Autodesk Inventor part; units mm, degrees
ref_plane "YZ Plane" through (0, 0, 0) normal (1, 0, 0) x (0, 1, 0)
ref_plane "XZ Plane" through (0, 0, 0) normal (0, 1, 0) x (-1, 0, 0)
ref_plane "XY Plane" through (0, 0, 0) normal (0, 0, 1) x (1, 0, 0)
sketch "Sketch1" plane through (0, 0, 0) normal (0, 0, 1) x (1, 0, 0)
  line L0 (-15, 12.5) -> (15, 12.5)
  line L1 (15, 12.5) -> (15, -12.5)
  line L2 (15, -12.5) -> (-15, -12.5)
  line L3 (-15, -12.5) -> (-15, 12.5)
  line L4 (-15, 12.5) -> (15, -12.5) construction
  line L5 (15, 12.5) -> (-15, -12.5) construction
  point P0 (0, 0)
  dimension "d0" = 30
  dimension "d1" = 25
extrude "Extrusion1" add sketch "Sketch1" along normal blind 30
sketch "Sketch2" plane through (15, -12.5, 0) normal (1, 0, 0) x (0, 0, -1)
  circle A0 centre (-15.0077, 12.5) radius 7.5
  point P0 (0, 12.5)
  dimension "d4" = 15
extrude "Extrusion2" cut sketch "Sketch2" against normal through all
sketch "Sketch3" plane through (-15, -12.5, 0) normal (0, -1, 0) x (1, 0, 0)
  line L0 (7.5, 23.9638) -> (22.5, 23.9638)
  line L1 (22.5, 23.9638) -> (22.5, 8.9638)
  line L2 (22.5, 8.9638) -> (7.5, 8.9638)
  line L3 (7.5, 8.9638) -> (7.5, 23.9638)
  line L4 (7.5, 23.9638) -> (22.5, 8.9638) construction
  line L5 (22.5, 23.9638) -> (7.5, 8.9638) construction
  point P0 (15, 0)
  point P1 (15, 16.4638)
  dimension "d7" = 15
  dimension "d8" = 15
extrude "Extrusion3" add sketch "Sketch3" along normal blind 25
sketch "Sketch4" plane through (-15, -37.5, 0) normal (0, -1, 0) x (1, 0, 0)
  line L0 (-0.1247, 34.0483) -> (29.8753, 34.0483)
  line L1 (29.8753, 34.0483) -> (29.8753, -0.9517)
  line L2 (29.8753, -0.9517) -> (-0.1247, -0.9517)
  line L3 (-0.1247, -0.9517) -> (-0.1247, 34.0483)
  line L4 (-0.1247, 34.0483) -> (29.8753, -0.9517) construction
  line L5 (29.8753, 34.0483) -> (-0.1247, -0.9517) construction
  point P0 (15, 0)
  point P1 (14.8753, 16.5483)
  dimension "d11" = 30
  dimension "d12" = 35
extrude "Extrusion4" add sketch "Sketch4" along normal blind 30
sketch "Sketch5" plane through (-15.1247, -37.5, -0.9517) normal (-1, 0, 0) x (0, 0, 1)
  circle A0 centre (17.4156, -15.0883) radius 7.5
  point P0 (0.9517, 37.5)
  dimension "d15" = 15
extrude "Extrusion5" add sketch "Sketch5" along normal blind 10
sketch "Sketch6" plane through (14.8753, -37.5, 34.0483) normal (1, 0, 0) x (0, 0, -1)
  circle A0 centre (17.5844, -15.0883) radius 7.5
  circle A1 centre (17.5844, -15.0883) radius 7.5
  point P0 (34.0483, 37.5)
extrude "Extrusion6" add sketch "Sketch6" along normal blind 10
sketch "Sketch7" plane through (-25.1247, -52.5883, 16.4638) normal (-1, 0, 0) x (0, 0, 1)
  line L0 (-17.4156, -14.9117) -> (17.5844, -14.9117)
  circle A0 centre (0, 0) radius 23.0558
  point P0 (-16.4638, 52.5883)
extrude "Extrusion7" add sketch "Sketch7" along normal blind 10
sketch "Sketch8" plane through (24.8753, -52.5883, 16.4638) normal (1, 0, 0) x (0, 0, -1)
  circle A0 centre (0, 0) radius 7.5
  circle A1 centre (0, 0) radius 23.0558
  circle A2 centre (0, 0) radius 23.056
  point P0 (16.4638, 52.5883)
  dimension "d22" = 46.112
extrude "Extrusion8" add sketch "Sketch8" along normal blind 10 contours A0 | A1
sketch "Sketch9" plane through (-15.1247, -37.5, 34.0483) normal (0, 0, 1) x (1, 0, 0)
  line L0 (2.6247, -2.5672) -> (27.6247, -2.5672)
  line L1 (27.6247, -2.5672) -> (27.6247, -27.5672)
  line L2 (27.6247, -27.5672) -> (2.6247, -27.5672)
  line L3 (2.6247, -27.5672) -> (2.6247, -2.5672)
  line L4 (2.6247, -2.5672) -> (27.6247, -27.5672) construction
  line L5 (27.6247, -2.5672) -> (2.6247, -27.5672) construction
  point P0 (15.1247, 37.5)
  point P1 (15.1247, -15.0672)
  dimension "d25" = 25
  dimension "d26" = 25
extrude "Extrusion9" cut sketch "Sketch9" against normal through all
properties part number "Part4f"
The model under review builds one solid part; all positions refer to its coordinate system, in mm. A direction names the side the tool comes from. Coordinates: 2 decimals unless noted, no trailing zeros. Write each loop counter-clockwise with the first axis right and the second up, starting at its lowest first coordinate (ties: lowest second). Pieces come first, ordered by that corner, then holes. Notation, with made-up numbers: (-36, -26) -> (-32, -26) arc R15 cw to (-32, 1) -> close; hole circle Ø7 at (-23, -32). An arc over 180 degrees is marked (long way). Answer in a Markdown table with one row per item.
1. We need section B-B, the plane x = 11.5. State the section outline as (y, z) points, and give its area (3 significant figures).
Answers below:
| item | result |
|---|---|
| outline | (-67.5, -0.95) -> (-65.07, -0.95) -> (-65.07, 34.05) -> (-67.5, 34.05) -> close; (-40.07, -0.95) -> (-37.5, -0.95) -> (-37.5, 34.05) -> (-40.07, 34.05) -> close; (-12.5, 0) -> (12.5, 0) -> (12.5, 30) -> (-12.5, 30) -> close; hole circle Ø15 at (0, 15.01) |
| area | 748 mm^2 |
2. Clearance check with flat-ended pins moving along their axes: pin 1 Ø12.5 at (y, z) = (2, 8.5) entering from -X; pin 2 Ø10 at (x, y) = (-8.5, -37.5) entering from -Z; pin 3 Ø2 at (x, z) = (1.5, 19) entering from -Y; pin 4 Ø15 at (x, y) = (3, -54.5) entering from +Z. State where each tip first meets the part, or that it passes through.
Answers below:
| item | result |
|---|---|
| pin 1 | stops at x = -15 |
| pin 2 | stops at z = -0.95 |
| pin 3 | stops at y = -67.5 |
| pin 4 | passes through |
3. We need section C-C, the plane z = 4. State the section outline as (x, y) points, and give its area (3 significant figures).
Answers below:
| item | result |
|---|---|
| outline | (-35.12, -71.98) -> (-25.12, -71.98) -> (-25.12, -33.19) -> (-35.12, -33.19) -> close; (-15.12, -67.5) -> (14.88, -67.5) -> (14.88, -37.5) -> (-15.12, -37.5) -> close; (-15, -12.5) -> (15, -12.5) -> (15, 12.5) -> (-15, 12.5) -> close; (24.88, -71.98) -> (34.88, -71.98) -> (34.88, -33.19) -> (24.88, -33.19) -> close; hole (-12.5, -65.07) -> (12.5, -65.07) -> (12.5, -40.07) -> (-12.5, -40.07) -> close |
| area | 1,800 mm^2 |
4. We need section D-D, the plane y = 0. State the section outline as (x, z) points.
Answers below:
| item | result |
|---|---|
| outline | (-15, 0) -> (15, 0) -> (15, 7.51) -> (-15, 7.51) -> close; (-15, 22.51) -> (15, 22.51) -> (15, 30) -> (-15, 30) -> close |
5. For faces 4 (the flat face through (15, 9, 15)), 5 (the flat face through (0, -40.067, 17)), 6 (the flat face through (-15, -9, 15)), 7 (the flat face through (0, -37.5, 25)), 8 (the flat face through (13, -52, -0.952)), list the 3-axis set-ups (+Z, -Z, +X, -X, +Y, -Y) from which the entire face can be reached by the end or side of a thin tool; tool diameter is ignored.
Answers below:
| item | result |
|---|---|
| face 4 | +Z, -Z, +X, +Y |
| face 5 | +Z, -Z |
| face 6 | +Z, -Z, -X, +Y |
| face 7 | none |
| face 8 | -Z, +Y, -Y |
6. Draft analysis for pull direction Z (two halves, no side actions). For faces 1 (the cylindrical face through (-30.055, -75.448, 13.462)), 2 (the flat face through (-25.125, -47, 11)), 3 (the cylindrical face through (0.21, -2.87, 8.08)), state which applies: +Z half, -Z half, draft (parallel to the pull), parting line (faces both ways), or undercut.
Answers below:
| item | result |
|---|---|
| face 1 | parting line |
| face 2 | draft |
| face 3 | undercut |
7. We need section A-A, the plane x = 3. State the section outline as (y, z) points.
Answers below:
| item | result |
|---|---|
| outline | (-67.5, -0.95) -> (-65.07, -0.95) -> (-65.07, 34.05) -> (-67.5, 34.05) -> close; (-40.07, -0.95) -> (-37.5, -0.95) -> (-37.5, 8.96) -> (-12.5, 8.96) -> (-12.5, 0) -> (12.5, 0) -> (12.5, 30) -> (-12.5, 30) -> (-12.5, 23.96) -> (-37.5, 23.96) -> (-37.5, 34.05) -> (-40.07, 34.05) -> close; hole circle Ø15 at (0, 15.01) |
8. Wall thickness on probe 1 along X at (y, z) = (-60, 28.5); probe 2 along X at (y, z) = (-54, 19.5); probe 3 along Y at (x, z) = (-6.5, 1): over which ranges is each line inside the solid? List them lowest first. Write a range as [from, to].
Answers below:
| item | result |
|---|---|
| probe 1 | x = [-35.12, -25.12], [-15.12, -12.5], [12.5, 14.88], [24.88, 34.88] |
| probe 2 | x = [-35.12, -12.5], [12.5, 34.88] |
| probe 3 | y = [-67.5, -65.07], [-40.07, -37.5], [-12.5, 12.5] |
